Check sheet for the modelled part. Datum: model origin and axes. Units: mm. Face numbers are marked on the shaded views. A direction names the side the tool comes from. Coordinates: 2 decimals unless noted, no trailing zeros. Loops run counter-clockwise (first coordinate to the right, second up) from the corner with the lowest first, then second, coordinate; pieces in that order, holes last. Notation, with made-up numbers: M 19,33 L 29,33 A23 cw 29,56 Z; hole C 86,29 d3. An arc over 180 degrees is marked long. Use CSV: the item, a comma, the result in double quotes. Start each with the question number.
(1) Scan lines: line 1 (Y direction, x = 0.5, z = 7.25); line 2 (Y direction, x = -0.5, z = 3); line 3 (Y direction, x = -20, z = -1.3). Record each from-to range of solid material in increasing order.
(2) Set-up check for the marked faces 1, 2, 3, 4 and 5: record each of +Z, -Z, +X, -X, +Y, -Y from which the full face is reachable in a straight line by a thin tool's end or side.
(3) Go/stop test with flat-tipped pins: pin 1 Ø0.7 at (x, z) = (5, 9) entering from +Y; pin 2 Ø2 at (x, y) = (0, 16.5) entering from +Z; pin 3 Ø2 at (x, z) = (-17, 10) entering from +Y. Record where each tip stops, or that it passes through.
(4) Section check D-D on x = -16. Record the cut outline in (y, z).
(5) Section check C-C on y = 22. Record the cut outline in (x, z), and give its area (3 significant figures).
(6) Section check A-A on z = 7.5. Record the cut outline in (x, y).
(7) Section check B-B on z = 1.25. Record the cut outline in (x, y).
(8) Draft check along Y on the marked faces 6, 7 and 8. Enter one of: pulls with the +Y half, pulls with the -Y half, needs draft (parallel to the pull), parting line crosses it, or undercut.
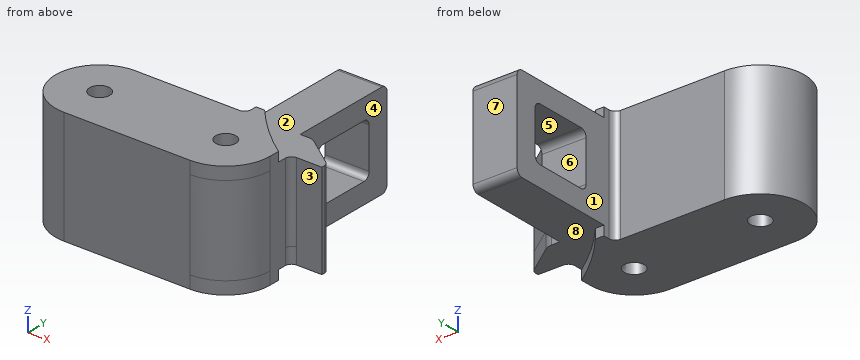
from build123d import *
from build123d.topology import SkipClean

# Parameters (mm, degrees)
SKETCH_1_R          = 7
SKETCH_1_R_2        = 1.6
EXTRUDE_1_DEPTH     = 14
FILLET_2_R          = 1
FILLET_4_R          = 2
FILLET_5_R          = 1
CUT_EXTRUDE_1_DEPTH = 10
SKETCH_4_R          = 43
SKETCH_4_W          = 56
SKETCH_4_H          = 56
CUT_EXTRUDE_2_DEPTH = 2
SKETCH_5_R          = 1.6
EXTRUDE_3_DEPTH     = 2
EXTRUDE_START       = 2
SKETCH_6_R          = 1.6
EXTRUDE_4_DEPTH     = 2
EXTRUDE_START_2     = 2.5
EXTRUDE_6_DEPTH     = 2.5
EXTRUDE_7_DEPTH     = 2.5
CUT_EXTRUDE_3_DEPTH = 43.558782877
SKETCH_15_W         = 6
SKETCH_15_H         = 15
EXTRUDE_10_DEPTH    = 1
EXTRUDE_START_3     = 1
SKETCH_14_W         = 15
SKETCH_14_H         = 17
EXTRUDE_9_DEPTH     = 1
FILLET_6_R          = 1


with BuildPart() as part:
    # 草图1 → 凸台-拉伸1 (new body)
    # profile 1 of 3: a face of its own
    with BuildSketch(Plane.XY):
        with BuildLine():
            Line((-2.5, 7), (-20, 7))
            ThreePointArc((-20, 7), (-15.050252532, 4.949747468), (-13, 0))
            ThreePointArc((-13, 0), (-15.050252532, -4.949747468), (-20, -7))
            Line((-20, -7), (0, -7))
            ThreePointArc((0, -7), (-4.949747468, 4.949747468), (7, 0))
            Line((7, 0), (7, 4))
            Line((7, 4), (12, 4))
            Line((12, 4), (12, 5))
            Line((12, 5), (6.5, 9))
            Line((6.5, 9), (3.5, 9))
            Line((3.5, 9), (3.5, 26))
            Line((3.5, 26), (-2.5, 26))
            Line((-2.5, 26), (-2.5, 7))
        make_face()
    # profile 2 of 3: a face of its own
    with BuildSketch(Plane.XY):
        Circle(SKETCH_1_R)
        Circle(SKETCH_1_R_2, mode=Mode.SUBTRACT)
    # profile 3 of 3: a face of its own
    with BuildSketch(Plane.XY):
        with Locations((-20, 0)):
            Circle(SKETCH_1_R)
        with Locations((-20, 0)):
            Circle(SKETCH_1_R_2, mode=Mode.SUBTRACT)
    extrude(amount=EXTRUDE_1_DEPTH)

    # 圆角2
    fillet_2_edges = [part.edges().sort_by_distance(p)[0] for p in [
        (-2.5, 7, 7),
        (7, 4, 7),
    ]]
    fillet(fillet_2_edges, radius=FILLET_2_R)

    # 圆角4
    fillet_4_edges = [part.edges().sort_by_distance(p)[0] for p in [
        (6.5, 9, 7),
    ]]
    fillet(fillet_4_edges, radius=FILLET_4_R)

    # 圆角5
    fillet_5_edges = [part.edges().sort_by_distance(p)[0] for p in [
        (12, 5, 7),
    ]]
    fillet(fillet_5_edges, radius=FILLET_5_R)

    # 草图2 → 切除-拉伸1 (cut)
    with BuildSketch(Plane(origin=(3.5, 0, 0), x_dir=(0, 0, -1), z_dir=(1, 0, 0))):
        Polygon((-12, 9), (-14, 9), (-14, 26), (0, 26), (0, 9), (-2, 9), (-2, 25), (-12, 25), align=None)
    extrude(amount=-CUT_EXTRUDE_1_DEPTH, mode=Mode.SUBTRACT)

    # 草图4 → 切除-拉伸2 (cut)
    with BuildSketch(Plane.XY.offset(14)):
        with Locations((31.5, 37)):
            Circle(SKETCH_4_R)
        with Locations((31.5, 37)):
            Rectangle(SKETCH_4_W, SKETCH_4_H, mode=Mode.SUBTRACT)
    cut_extrude_2 = extrude(amount=-CUT_EXTRUDE_2_DEPTH, mode=Mode.SUBTRACT)

    # 镜向1: 切除-拉伸2 across plane
    add(cut_extrude_2.mirror(Plane.XY.offset(7)), mode=Mode.SUBTRACT)

    # 草图5 → 凸台-拉伸3 (add)
    with SkipClean():  # the faces are left unmerged after this step: merging them gives an invalid solid
        with BuildSketch(Plane.XY.offset(14)):
            with BuildLine():
                Line((-1.134337744, 9), (-2.5, 9))
                Line((-2.5, 9), (-2.5, 8))
                ThreePointArc((-2.5, 8), (-2.792893219, 7.292893219), (-3.5, 7))
                Line((-3.5, 7), (-20, 7))
                ThreePointArc((-20, 7), (-27, 0), (-20, -7))
                Line((-20, -7), (0, -7))
                ThreePointArc((0, -7), (4.949747468, -4.949747468), (7, 0))
                Line((7, 0), (7, 1.662343032))
                ThreePointArc((7, 1.662343032), (2.698204226, 5.071070168), (-1.134337744, 9))
            make_face()
            Circle(SKETCH_5_R, mode=Mode.SUBTRACT)
            with Locations((-20, 0)):
                Circle(SKETCH_5_R, mode=Mode.SUBTRACT)
        extrude(amount=EXTRUDE_3_DEPTH)

    # 草图6 → 凸台-拉伸4 (add)
    with SkipClean():  # the faces are left unmerged after this step: merging them gives an invalid solid
        with BuildSketch(Plane(origin=(0, 0, 0), x_dir=(-1, 0, 0), z_dir=(0, 0, -1)).offset(EXTRUDE_START)):
            with BuildLine():
                Line((-7, 1.662343032), (-7, 0))
                ThreePointArc((-7, 0), (-4.949747468, -4.949747468), (0, -7))
                Line((0, -7), (20, -7))
                ThreePointArc((20, -7), (27, 0), (20, 7))
                Line((20, 7), (3.5, 7))
                ThreePointArc((3.5, 7), (2.792893219, 7.292893219), (2.5, 8))
                Line((2.5, 8), (2.5, 9))
                Line((2.5, 9), (1.134337744, 9))
                ThreePointArc((1.134337744, 9), (-2.698204226, 5.071070168), (-7, 1.662343032))
            make_face()
            with Locations((20, 0)):
                Circle(SKETCH_6_R, mode=Mode.SUBTRACT)
            Circle(SKETCH_6_R, mode=Mode.SUBTRACT)
        extrude(amount=-EXTRUDE_4_DEPTH)

    # 草图8 → 凸台-拉伸6 (add)
    with BuildSketch(Plane.XY.offset(12).offset(EXTRUDE_START_2)):
        with BuildLine():
            Line((-2.5, 9), (-1.134337744, 9))
            ThreePointArc((-1.134337744, 9), (2.698204226, 5.071070168), (7, 1.662343032))
            Line((7, 1.662343032), (7, 3))
            ThreePointArc((7, 3), (7.292893219, 3.707106781), (8, 4))
            Line((8, 4), (12, 4))
            Line((12, 4), (12, 4.490775408))
            ThreePointArc((12, 4.490775408), (11.891114947, 4.944553053), (11.588171698, 5.299511493))
            Line((11.588171698, 5.299511493), (7.025975768, 8.617472169))
            ThreePointArc((7.025975768, 8.617472169), (6.468120717, 8.901965344), (5.849632373, 9))
            Line((5.849632373, 9), (3.5, 9))
            Line((3.5, 9), (3.5, 25))
            Line((3.5, 25), (-2.5, 25))
            Line((-2.5, 25), (-2.5, 9))
        make_face()
    extrude(amount=-EXTRUDE_6_DEPTH)

    # 草图9 → 凸台-拉伸7 (add)
    with BuildSketch(Plane(origin=(0, 0, 2), x_dir=(-1, 0, 0), z_dir=(0, 0, -1))):
        with BuildLine():
            Line((-3.5, 25), (-3.5, 9))
            Line((-3.5, 9), (-5.849632373, 9))
            ThreePointArc((-5.849632373, 9), (-6.468120717, 8.901965344), (-7.025975768, 8.617472169))
            Line((-7.025975768, 8.617472169), (-11.588171698, 5.299511493))
            ThreePointArc((-11.588171698, 5.299511493), (-11.891114947, 4.944553053), (-12, 4.490775408))
            Line((-12, 4.490775408), (-12, 4))
            Line((-12, 4), (-8, 4))
            ThreePointArc((-8, 4), (-7.292893219, 3.707106781), (-7, 3))
            Line((-7, 3), (-7, 1.662343032))
            ThreePointArc((-7, 1.662343032), (-2.698204226, 5.071070168), (1.134337744, 9))
            Line((1.134337744, 9), (2.5, 9))
            Line((2.5, 9), (2.5, 25))
            Line((2.5, 25), (-3.5, 25))
        make_face()
    extrude(amount=EXTRUDE_7_DEPTH)

    # 草图13 → 切除-拉伸3 (cut, through all)
    with BuildSketch(Plane(origin=(3.5, 0, 0), x_dir=(0, 0, -1), z_dir=(1, 0, 0))):
        with BuildLine():
            Line((-10.25, 22.5), (-3.75, 22.5))
            ThreePointArc((-3.75, 22.5), (-3.042893219, 22.207106781), (-2.75, 21.5))
            Line((-2.75, 21.5), (-2.75, 13.5))
            ThreePointArc((-2.75, 13.5), (-3.042893219, 12.792893219), (-3.75, 12.5))
            Line((-3.75, 12.5), (-10.25, 12.5))
            ThreePointArc((-10.25, 12.5), (-10.957106781, 12.792893219), (-11.25, 13.5))
            Line((-11.25, 13.5), (-11.25, 21.5))
            ThreePointArc((-11.25, 21.5), (-10.957106781, 22.207106781), (-10.25, 22.5))
        make_face()
    extrude(amount=-CUT_EXTRUDE_3_DEPTH, mode=Mode.SUBTRACT)

    # 草图15 → 凸台-拉伸10 (add)
    with BuildSketch(Plane(origin=(0, 25, 0), x_dir=(1, 0, 0), z_dir=(0, 1, 0))):
        with Locations((0.5, -7)):
            Rectangle(SKETCH_15_W, SKETCH_15_H)
    extrude(amount=EXTRUDE_10_DEPTH)

    # 草图14 → 凸台-拉伸9 (add)
    with BuildSketch(Plane(origin=(3.5, 0, 0), x_dir=(0, 0, -1), z_dir=(1, 0, 0)).offset(EXTRUDE_START_3)):
        with Locations((-7, 17.5)):
            Rectangle(SKETCH_14_W, SKETCH_14_H)
        with BuildLine():
            Line((-2.75, 13.5), (-2.75, 21.5))
            ThreePointArc((-2.75, 21.5), (-3.042893219, 22.207106781), (-3.75, 22.5))
            Line((-3.75, 22.5), (-10.25, 22.5))
            ThreePointArc((-10.25, 22.5), (-10.957106781, 22.207106781), (-11.25, 21.5))
            Line((-11.25, 21.5), (-11.25, 13.5))
            ThreePointArc((-11.25, 13.5), (-10.957106781, 12.792893219), (-10.25, 12.5))
            Line((-10.25, 12.5), (-3.75, 12.5))
            ThreePointArc((-3.75, 12.5), (-3.042893219, 12.792893219), (-2.75, 13.5))
        make_face(mode=Mode.SUBTRACT)
    extrude(amount=-EXTRUDE_9_DEPTH)

    # 圆角6
    fillet_6_edges = [part.edges().sort_by_distance(p)[0] for p in [
        (1, 26, -0.5),
        (1, 26, 14.5),
    ]]
    fillet(fillet_6_edges, radius=FILLET_6_R)


solid = part.part
Outcome:
1,line 1,"y = -6.98 to -1.52, 1.52 to 12.5, 22.5 to 26"
1,line 2,"y = -7 to -1.52, 1.52 to 12.84, 22.16 to 26"
1,line 3,"y = -7 to -1.6, 1.6 to 7"
2,face 1,"+Z, -Z, -X, +Y"
2,face 2,"+Z, +X, +Y"
2,face 3,"+Z, -Z, +X, -Y"
2,face 4,"+Z, -Z, +X, +Y"
2,face 5,"+X, -X"
3,pin 1,"stops at y = 9"
3,pin 2,"stops at z = 14.5"
3,pin 3,"stops at y = 7"
4,outline,"M -7,-2 L 7,-2 L 7,16 L -7,16 Z"
5,outline,"M -2.5,-0.5 L 4.5,-0.5 L 4.5,2.88 L -2.5,2.88 Z; M -2.5,11.12 L 4.5,11.12 L 4.5,14.5 L -2.5,14.5 Z"
5,area,"47.4 mm²"
6,outline,"M -20,-7 L 0,-7 A7 ccw 7,0 L 7,3 A1 cw 8,4 L 12,4 L 12,4.49 A1 ccw 11.59,5.3 L 7.03,8.62 A2 ccw 5.85,9 L 4.5,9 L 4.5,12.5 L -2.5,12.5 L -2.5,8 A1 cw -3.5,7 L -20,7 A7 ccw Z; M -2.5,22.5 L 4.5,22.5 L 4.5,26 L -2.5,26 Z; hole C -20,0 d3.2; hole C 0,0 d3.2"
7,outline,"M -20,-7 L 0,-7 A7 ccw 7,0 L 7,3 A1 cw 8,4 L 12,4 L 12,4.49 A1 ccw 11.59,5.3 L 7.03,8.62 A2 ccw 5.85,9 L 4.5,9 L 4.5,26 L -2.5,26 L -2.5,8 A1 cw -3.5,7 L -20,7 A7 ccw Z; hole C -20,0 d3.2; hole C 0,0 d3.2"
8,face 6,"undercut"
8,face 7,"pulls with the +Y half"
8,face 8,"needs draft"
